```python
from build123d import *

# Parameters (mm, degrees)
SKETCH1_R           = 12.7
BOSS_EXTRUDE1_DEPTH = 77.978
SKETCH2_R           = 4.7625
BOSS_EXTRUDE2_DEPTH = 19.812
FILLET1_R           = 7.62


with BuildPart() as part:
    # Sketch1 → Boss-Extrude1 (new body)
    with BuildSketch(Plane(origin=(0, 0, 0), x_dir=(1, 0, 0), z_dir=(0, 1, 0))):
        with Locations(Location((0, 0, 0), (0, 0, 270))):
            Circle(SKETCH1_R)
    extrude(amount=BOSS_EXTRUDE1_DEPTH)

    # Sketch2 → Boss-Extrude2 (add)
    with BuildSketch(Plane(origin=(0, 77.978, 0), x_dir=(1, 0, 0), z_dir=(0, 1, 0))):
        with Locations(Location((0, 0, 0), (0, 0, 270))):
            Circle(SKETCH2_R)
    boss_extrude2 = extrude(amount=BOSS_EXTRUDE2_DEPTH)

    # Mirror1: Boss-Extrude2 across plane
    add(boss_extrude2.mirror(Plane.ZX.offset(38.989)))

    # Fillet1
    fillet1_edges = [part.edges().sort_by_distance(p)[0] for p in [
        (0, 0, -4.7625),
        (0, 77.978, -4.7625),
    ]]
    fillet(fillet1_edges, radius=FILLET1_R)


solid = part.part
```
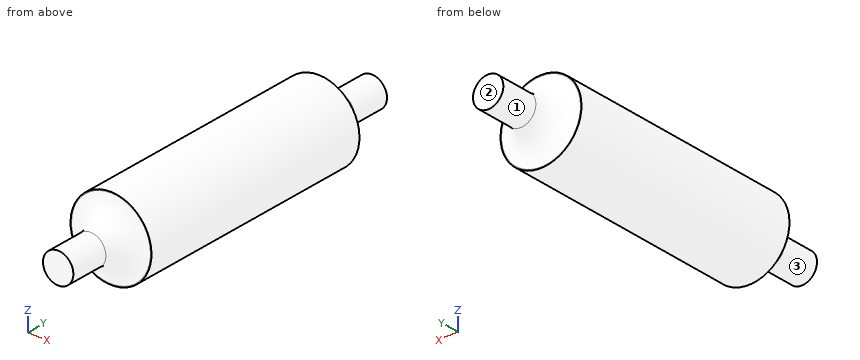
Check sheet for the modelled part. Datum: model origin and axes. Units: mm. Face numbers are marked on the shaded views. A direction names the side the tool comes from. Coordinates: 2 decimals unless noted, no trailing zeros. Loops run counter-clockwise (first coordinate to the right, second up) from the corner with the lowest first, then second, coordinate; pieces in that order, holes last.
1) Sectioned sample at A-A (z = 0). Record the boundary of the cut face in (x, y), and give its area (3 significant figures).
2) Access from +Z, -Z, +X, -X, +Y, -Y to the whole of each face (thin tool, end or side, straight path). Record for the marked faces 1, 2 and 3.
3) Material ranges on probe 1 along X at (y, z) = (70, 2.75); probe 2 along X at (y, z) = (73.5, 0.5); probe 3 along Z at (x, y) = (0.25, 56), recorded low to high.
4) Gauge pin test, flat ends, axial feed: pin 1 (5 mm diameter, centred on y = 29.5, z = -8, fed in from +X); pin 2 (1 mm diameter, centred on x = 6, y = 24.5, fed in from -Z); pin 3 (1 mm diameter, centred on x = -2.5, y = 39, fed in from -Z). Record the tip position at first contact, or that the pin passes through.
5) Sectioned sample at B-B (x = 0). Record the boundary of the cut face in (y, z), and give its area (3 significant figures).
Check sheet entries:
1. outline: (-12.7, 0) - (-12.38, 0) arc R7.62 cw to (-4.76, -7.62) - (-4.76, -19.81) - (4.76, -19.81) - (4.76, -7.62) arc R7.62 cw to (12.38, 0) - (12.7, 0) - (12.7, 77.98) - (12.38, 77.98) arc R7.62 cw to (4.76, 85.6) - (4.76, 97.79) - (-4.76, 97.79) - (-4.76, 85.6) arc R7.62 cw to (-12.38, 77.98) - (-12.7, 77.98) - close
1. area: 2,410 mm2
2. face 1: +Y
2. face 2: +Z, -Z, +X, -X, +Y
2. face 3: -Y
3. probe 1: x = -12.4 to 12.4
3. probe 2: x = -12.69 to 12.69
3. probe 3: z = -12.7 to 12.7
4. pin 1: stops at x = 11.45
4. pin 2: stops at z = -11.45
4. pin 3: stops at z = -12.54
5. outline: (-19.81, -4.76) - (-7.62, -4.76) arc R7.62 cw to (0, -12.38) - (0, -12.7) - (77.98, -12.7) - (77.98, -12.38) arc R7.62 cw to (85.6, -4.76) - (97.79, -4.76) - (97.79, 4.76) - (85.6, 4.76) arc R7.62 cw to (77.98, 12.38) - (77.98, 12.7) - (0, 12.7) - (0, 12.38) arc R7.62 cw to (-7.62, 4.76) - (-19.81, 4.76) - close
5. area: 2,410 mm2
